Check sheet for the modelled part. Datum: model origin and axes. Units: mm. A direction names the side the tool comes from. Give positions to 0.01 mm unless a question says otherwise; leave off trailing zeros. Loops run counter-clockwise (first coordinate to the right, second up) from the corner with the lowest first, then second, coordinate; pieces in that order, holes last. Notation, with made-up numbers: (72, -21.5) -> (126, -21.5) arc R13 ccw to (126, -6.5) -> close; hole circle Ø4 at (-35, 43). An arc over 180 degrees is marked (long way). Write each question's results on one line, items separated by ' | '. Start each with the question number.
Item 1: Gauge pin test, flat ends, axial feed: pin 1 Ø1 at (x, y) = (19.5, -3) entering from +Z; pin 2 Ø1.8 at (y, z) = (-1.5, -78) entering from +X; pin 3 Ø1 at (y, z) = (-1, -84.5) entering from -X. Record the tip position at first contact, or that the pin passes through.
Item 2: Access from +Z, -Z, +X, -X, +Y, -Y to the whole of each face (thin tool, end or side, straight path). Record for faces 5 (the face through (-23.235, -2, -12)), 6 (the face through (-9, -3.556, -25)).
Item 3: Cross-section at B-B on z = -10. Enter the section's corners in (x, y).
Item 4: Scan lines: line 1 along X through (y, z) = (-2.65, -92); line 2 along X through (y, z) = (-2, -70); line 3 along Z through (x, y) = (-16, -3.4). Record each from-to range of solid material in increasing order.
Item 5: Cross-section at C-C on x = 21.5. Enter the section's corners in (y, z), then the cut area to 3 significant figures.
Item 6: Cross-section at A-A on y = -2. Enter the section's corners in (x, z).
Item 7: Mould release check, pull along X, two halves, no side actions. Record for faces 1 (the face through (-23.235, -2, -113)), 2 (the face through (-15, -2, -156.524)), 3 (the face through (-5.826, -2, -83)), 4 (the face through (28.963, -1.753, 2.231)): pulls with the +X half, pulls with the -X half, needs draft (parallel to the pull), parting line crosses it, or undercut.
from build123d import *

# Parameters (mm, degrees)
F1_DEPTH = 3.556


with BuildPart() as f1:
    # F0 (on Front) → F1 (new body)
    with BuildSketch(Plane.XZ):
        with BuildLine():
            Line((-5.826374, -156.523644), (-5.826374, -7.032426))
            ThreePointArc((-5.826374, -7.032426), (1.871411, -3.572466), (8.417938, 1.753902))
            ThreePointArc((8.417938, 1.753902), (29.123373, 2.547832), (16.949844, 19.315377))
            ThreePointArc((16.949844, 19.315377), (-33.159966, 51.122593), (-23.235221, -7.393999))
            Line((-23.235221, -7.393999), (-23.235221, -16.009105))
            Line((-23.235221, -16.009105), (-24.5104, -16.009105))
            Line((-24.5104, -16.009105), (-23.943633, -71.23325))
            Line((-23.943633, -71.23325), (-23.235221, -71.23325))
            Line((-23.235221, -71.23325), (-23.235221, -140.258765))
            Line((-23.235221, -140.258765), (-23.235221, -156.523644))
            Line((-23.235221, -156.523644), (-5.826374, -156.523644))
        make_face()
    extrude(amount=F1_DEPTH)


solid = f1.part
Answer sheet:
1) pin 1: stops at z = 19.42 | pin 2: stops at x = -5.83 | pin 3: stops at x = -23.24
2) face 5: -X, +Y, -Y | face 6: +Z, -Z, +X, -X, -Y
3) outline: (-23.24, -3.56) -> (-5.83, -3.56) -> (-5.83, 0) -> (-23.24, 0) -> close
4) line 1: x = -23.24 to -5.83 | line 2: x = -23.96 to -5.83 | line 3: z = -156.52 to 56.54
5) outline: (-3.56, -3.69) -> (0, -3.69) -> (0, 19.05) -> (-3.56, 19.05) -> close | area: 80.9 mm²
6) outline: (-24.51, -16.01) -> (-23.94, -71.23) -> (-23.24, -71.23) -> (-23.24, -156.52) -> (-5.83, -156.52) -> (-5.83, -7.03) arc R32.48 ccw to (8.42, 1.75) arc R11.75 ccw (long way) to (16.95, 19.32) arc R32.48 ccw (long way) to (-23.24, -7.39) -> (-23.24, -16.01) -> close
7) face 1: pulls with the -X half | face 2: needs draft | face 3: pulls with the +X half | face 4: undercut
